```python
from build123d import *

# Parameters (mm, degrees)
F0_R     = 11.1
F1_DEPTH = 7
F2_R     = 5
F3_R     = 2


with BuildPart() as f1:
    # F0 (on Top) → F1 (new body)
    with BuildSketch(Plane.XY):
        with BuildLine():
            ThreePointArc((12.5, 8.291562), (0, 15), (-12.5, 8.291562))
            ThreePointArc((-12.5, 8.291562), (-40, 0), (-12.5, -8.291562))
            ThreePointArc((-12.5, -8.291562), (0, -15), (12.5, -8.291562))
            ThreePointArc((12.5, -8.291562), (40, 0), (12.5, 8.291562))
        make_face()
        with Locations((-25, 0)):
            Circle(F0_R, mode=Mode.SUBTRACT)
        Circle(F0_R, mode=Mode.SUBTRACT)
        with Locations((25, 0)):
            Circle(F0_R, mode=Mode.SUBTRACT)
    extrude(amount=F1_DEPTH)

    # F2
    f2_edges = [f1.edges().sort_by_distance(p)[0] for p in [
        (-12.5, -8.291562, 3.5),
        (12.5, -8.291562, 3.5),
        (12.5, 8.291562, 3.5),
        (-12.5, 8.291562, 3.5),
    ]]
    fillet(f2_edges, radius=F2_R)

    # F3
    f3_edges = [f1.edges().sort_by_distance(p)[0] for p in [
        (-40, 0, 7),
        (-40, 0, 0),
    ]]
    fillet(f3_edges, radius=F3_R)


solid = f1.part
```
Geometry check sheet. Reference: the model listing, model coordinates, mm. Round coordinates to 2 decimals unless told otherwise and drop trailing zeros. Loops run counter-clockwise (first coordinate to the right, second up) from the corner with the lowest first, then second, coordinate; pieces in that order, holes last. Notation, with made-up numbers: (-17, 74) - (11, 74) arc R26 cw to (11, 112) - close; hole circle Ø10 at (48, 54). An arc over 180 degrees is marked (long way). Use a Markdown table: item, result.
Q1. Draft check along X on faces 1 (the flat face through (11.1, 2, 7)), 2 (the cylindrical face through (5.97, 9.36, 3.45)). Enter one of: released by +X, released by -X, zero draft, split by the parting line, or undercut.
Solutions:
| item | result |
|---|---|
| face 1 | zero draft |
| face 2 | undercut |
Q2. Cross-section at C-C on z = 1. State how many separate pieces and enclosed holes the cut face has, plus the area to 3 significant figures.
Solutions:
| item | result |
|---|---|
| separate pieces | 1 |
| enclosed holes | 3 |
| area | 812 mm2 |
Q3. Material ranges on line 1 (X direction, y = -0.5, z = 3.25); line 2 (Y direction, x = 24.5, z = 4.25); line 3 (X direction, y = 11.5, z = 4.75), recorded low to high.
Solutions:
| item | result |
|---|---|
| line 1 | x = -39.99 to -36.09, -13.91 to -11.09, 11.09 to 13.91, 36.09 to 39.99 |
| line 2 | y = -14.99 to -11.09, 11.09 to 14.99 |
| line 3 | x = -34.63 to -15.34, -9.66 to 9.66, 15.34 to 34.63 |
Q4. Go/stop test with flat-tipped pins: P1, Ø1.5, axis at y = -5, z = 6.5, coming from the -X side; P2, Ø2, axis at y = 2, z = 3.5, coming from the +X side; P3, Ø1.5, axis at x = -20.5, z = 2.5, coming from the -Y side. Record where each tip stops, or that it passes through.
Solutions:
| item | result |
|---|---|
| P1 | stops at x = -39.07 |
| P2 | stops at x = 39.97 |
| P3 | stops at y = -14.52 |
Q5. Cross-section at A-A on y = 0. Record the cut outline in (x, z), plus the area to 3 significant figures.
Solutions:
| item | result |
|---|---|
| outline | (-40, 2) arc R2 ccw to (-38, 0) - (-36.1, 0) - (-36.1, 7) - (-38, 7) arc R2 ccw to (-40, 5) - close; (-13.9, 0) - (-11.1, 0) - (-11.1, 7) - (-13.9, 7) - close; (11.1, 0) - (13.9, 0) - (13.9, 7) - (11.1, 7) - close; (36.1, 0) - (38, 0) arc R2 ccw to (40, 2) - (40, 5) arc R2 ccw to (38, 7) - (36.1, 7) - close |
| area | 90.4 mm2 |
Q6. Cross-section at B-B on x = 0. Record the cut outline in (y, z).
Solutions:
| item | result |
|---|---|
| outline | (-15, 2) arc R2 ccw to (-13, 0) - (-11.1, 0) - (-11.1, 7) - (-13, 7) arc R2 ccw to (-15, 5) - close; (11.1, 0) - (13, 0) arc R2 ccw to (15, 2) - (15, 5) arc R2 ccw to (13, 7) - (11.1, 7) - close |
